```python
from build123d import *

# Parameters (mm, degrees)
BOSS_EXTRUDE2_DEPTH     = 125
CUT_EXTRUDE1_DEPTH      = 225.548075315
CUT_EXTRUDE1_DEPTH_BACK = 225.548075315
SKETCH9_R               = 20


with BuildPart() as part:
    # Sketch7 → Boss-Extrude2 (new, symmetric)
    with BuildSketch(Plane(origin=(0, 0, 0), x_dir=(0, 0, -1), z_dir=(1, 0, 0))):
        Polygon((0, 6.47), (-40, 6.47), (-40, 181.47), (-23.039187078, 181.47), align=None)
    extrude(amount=BOSS_EXTRUDE2_DEPTH, both=True)

    # Sketch9 → Cut-Extrude1 (cut, two sides: drawn at the far end of the back side and taken through both)
    with BuildSketch(Plane(origin=(0, 0.893387105, -6.785948779), x_dir=(-1, 0, 0), z_dir=(0, 0.130526192220056, -0.9914448613738098)).offset(-CUT_EXTRUDE1_DEPTH_BACK)):
        with Locations(Location((0, 127.16, 0), (0, 0, 90))):
            Circle(SKETCH9_R)
    extrude(amount=CUT_EXTRUDE1_DEPTH + CUT_EXTRUDE1_DEPTH_BACK, mode=Mode.SUBTRACT)


solid = part.part
```
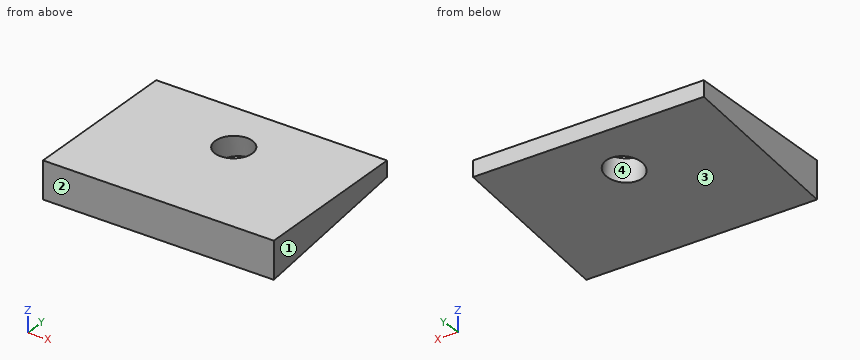
Verification items for the finished model (mm, model axes). Face numbers are marked on the shaded views. Give positions to 0.01 mm unless a question says otherwise; leave off trailing zeros. Loops run counter-clockwise (first coordinate to the right, second up) from the corner with the lowest first, then second, coordinate; pieces in that order, holes last. Notation, with made-up numbers: M 18,-7 L 35,-7 A12 cw 35,-1 Z; hole C 27.25,38 d6. An arc over 180 degrees is marked long. Return JSON: item names as keys, results as strings.
1) Mould release check, pull along Y, two halves, no side actions. Record for the marked faces 1, 2, 3 and 4: released by +Y, released by -Y, zero draft, split by the parting line, or undercut.
Findings:
{"face 1": "zero draft", "face 2": "released by -Y", "face 3": "released by +Y", "face 4": "undercut"}
2) Section check A-A, the plane x = 87. Enter the section's corners in (y, z).
Findings:
{"outline": "M 6.47,0 L 181.47,23.04 L 181.47,40 L 6.47,40 Z"}
3) Material ranges on L1, parallel to Y at x = 17, z = 36; L2, parallel to Y at x = -9, z = 24; L3, parallel to Z at x = 98, y = 86, recorded low to high. Write a range as [from, to].
Findings:
{"L1": "y = [6.47, 112.89], [134.14, 181.47]", "L2": "y = [6.47, 107.08], [143.11, 181.47]", "L3": "z = [10.47, 40]"}
4) Section check B-B, the plane y = 169.5. Enter the section's corners in (x, z), and give its area (3 significant figures).
Findings:
{"outline": "M -125,21.46 L 125,21.46 L 125,40 L -125,40 Z", "area": "4,630 mm2"}
5) Gauge pin test, flat end, axial feed: P1, Ø12, axis at x = -46.5, y = 31, coming from the -Z side. Record the tip position at first contact, or that the pin passes through.
Findings:
{"P1": "stops at z = 2.44"}
